For this review, take the finished solid that the model builds, in its own axes (mm). Round coordinates to 2 decimals unless told otherwise and drop trailing zeros. Order: outer loops, then holes, each group sorted by start corner. A loop starts at its lowest first (then second) coordinate and runs counter-clockwise, first axis right, second up.
Autodesk Inventor part; units mm, degrees
ref_plane "YZ Plane" through (0, 0, 0) normal (1, 0, 0) x (0, 1, 0)
ref_plane "XZ Plane" through (0, 0, 0) normal (0, 1, 0) x (-1, 0, 0)
ref_plane "XY Plane" through (0, 0, 0) normal (0, 0, 1) x (1, 0, 0)
sketch "Sketch1" plane through (0, 0, 0) normal (0, 1, 0) x (-1, 0, 0)
  line L0 (0, 0) -> (170, 0)
  line L1 (170, 0) -> (170, -220)
  line L2 (170, -220) -> (0, -220)
  line L3 (0, -220) -> (0, 0)
  dimension "d0" = 170
  dimension "d1" = 220
extrude "base" add sketch "Sketch1" along normal blind 2
chamfer "chamfers" distance 2 angle 45 2 edges at (-170, 2, -110) (0, 2, -110)
sketch "holes" plane through (0, 2, 0) normal (0, 1, 0) x (1, 0, 0)
  line L0 (-170, 220) -> (-170, 0)
  line L1 (0, 220) -> (-170, 220)
  line L2 (-170, 0) -> (0, 0)
  line L3 (0, 0) -> (0, 220)
  line L4 (0, 220) -> (-170, 220)
  line L5 (-170, 220) -> (-170, 0)
  line L6 (-168, 45) -> (-2, 45)
  line L7 (-2, 45) -> (-2, 175)
  line L8 (-2, 175) -> (-168, 175)
  line L9 (-168, 175) -> (-168, 45)
  line L10 (-2, 45) -> (-8, 45)
  line L11 (-8, 45) -> (-8, 51)
  line L12 (-8, 51) -> (-2, 51)
  line L13 (-2, 51) -> (-2, 45)
  line L14 (-2, 175) -> (-8, 175)
  line L15 (-8, 175) -> (-8, 169)
  line L16 (-8, 169) -> (-2, 169)
  line L17 (-2, 169) -> (-2, 175)
  line L18 (-168, 45) -> (-162, 45)
  line L19 (-162, 45) -> (-162, 51)
  line L20 (-162, 51) -> (-168, 51)
  line L21 (-168, 51) -> (-168, 45)
  line L22 (-168, 175) -> (-162, 175)
  line L23 (-162, 175) -> (-162, 169)
  line L24 (-162, 169) -> (-168, 169)
  line L25 (-168, 169) -> (-168, 175)
  point P0 (-85, 175)
  point P1 (-85, 220)
  point P2 (-168, 110)
  point P3 (-170, 110)
  point P4 (-165, 48)
  point P5 (-165, 172)
  point P6 (-5, 172)
  point P7 (-5, 48)
  point P8 (-85, 110)
  dimension "d10" = 166
  dimension "d11" = 130
  dimension "d12" = 6
  dimension "d13" = 6
  dimension "d14" = 6
  dimension "d15" = 6
  dimension "d16" = 6
  dimension "d17" = 6
  dimension "d18" = 6
hole "magnet_holders" at (-165, 2, -48) at (-165, 2, -172) at (-5, 2, -172) at (-5, 2, -48) direction (0, -1, 0) diameter 5.5 depth 1
hole "wire_hole" at (-85, 2, -110) direction (0, -1, 0) diameter 30 end through all
properties part number "lid"
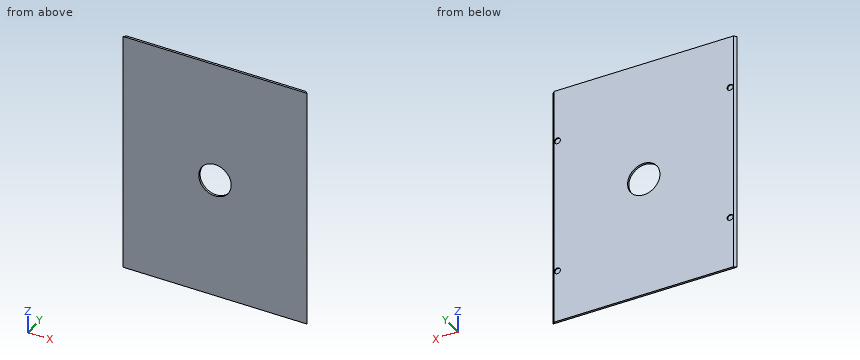
Q1. Take a section at D-D, the plane x = -5. State the section outline as (y, z) points, plus the area to 3 significant figures.
Q2. Take a section at A-A, the plane x = -85. State the section outline as (y, z) points.
Q3. Wall thickness on line 1 (Z direction, x = -165, y = 1.35); line 2 (X direction, y = 1.2, z = -48); line 3 (Z direction, x = -85, y = 1.4): over which ranges is each line inside the solid? List them lowest first.
Q4. Clearance check with a flat-ended pin moving along its axis: pin 1 (3 mm diameter, centred on x = -166, z = -47.5, fed in from +Y). State where the tip first meets the part, or that it passes through.
Working result:
1. outline: (0, -220) - (2, -220) - (2, -174.75) - (1, -174.75) - (1, -169.25) - (2, -169.25) - (2, -50.75) - (1, -50.75) - (1, -45.25) - (2, -45.25) - (2, 0) - (0, 0) - close
1. area: 429 mm2
2. outline: (0, -220) - (2, -220) - (2, -125) - (0, -125) - close; (0, -95) - (2, -95) - (2, 0) - (0, 0) - close
3. line 1: z = -220 to -174.75, -169.25 to -50.75, -45.25 to 0
3. line 2: x = -168.8 to -167.75, -162.25 to -7.75, -2.25 to -1.2
3. line 3: z = -220 to -125, -95 to 0
4. pin 1: stops at y = 1
